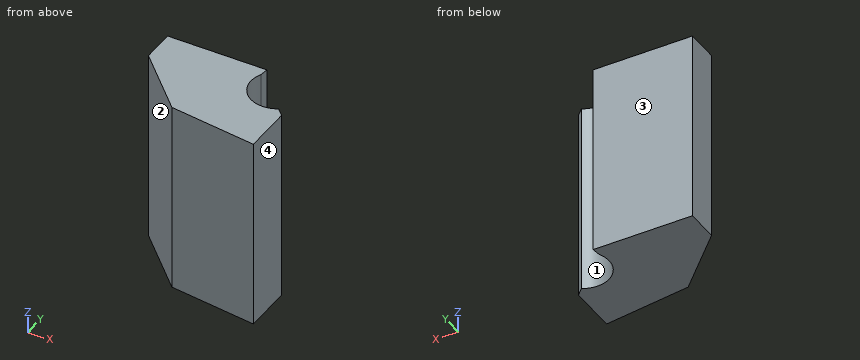
```python
from build123d import *

# Parameters (mm, degrees)
BOSS_EXTRU_1_DEPTH = 60
CHANFREIN1_START   = -1
CHANFREIN1_DEPTH   = 62
CHANFREIN2_SIZE    = 15
CHANFREIN2_SIZE2   = 17.409920551


with BuildPart() as part:
    # Esquisse1 → Boss.-Extru.1 (new body)
    with BuildSketch(Plane.XY):
        with BuildLine():
            Line((-1.739730228, 1.739730228), (-46.4022226, 7.592964471))
            Line((-46.4022226, 7.592964471), (-46.4022226, 32.915406071))
            Line((-46.4022226, 32.915406071), (-13.716955803, 32.915406071))
            ThreePointArc((-13.716955803, 32.915406071), (-14.250137868, 20.404998431), (-1.739730228, 20.938180496))
            Line((-1.739730228, 20.938180496), (-1.739730228, 1.739730228))
        make_face()
    extrude(amount=BOSS_EXTRU_1_DEPTH)

    # Chanfrein1: read off the stored shape, not the designer's step
    # Chanfrein1 outline → Chanfrein1 (cut)
    with BuildSketch(Plane.XY.offset(CHANFREIN1_START)):
        with BuildLine():
            ThreePointArc((-1.739730228, 20.938180496), (-2.7453552, 19.929895832), (-3.905196789, 19.103647058))
            Line((-3.905196789, 19.103647058), (-1.739730228, 16.938180496))
            Line((-1.739730228, 16.938180496), (-1.739730228, 20.938180496))
        make_face()
        with BuildLine():
            Line((-15.530475388, 32.915406071), (-15.835720777, 30.229973881))
            ThreePointArc((-15.835720777, 30.229973881), (-14.912820327, 31.680372218), (-13.716955803, 32.915406071))
            Line((-13.716955803, 32.915406071), (-15.530475388, 32.915406071))
        make_face()
    extrude(amount=CHANFREIN1_DEPTH, mode=Mode.SUBTRACT)

    # Chanfrein2
    chanfrein2_edges = [part.edges().sort_by_distance(p)[0] for p in [
        (-46.4022226, 7.592964471, 30),
    ]]
    chanfrein2_side = [part.faces().sort_by_distance(p)[0] for p in [
        (-46.4022226, 20.254185271, 30),
    ]]
    chamfer(chanfrein2_edges, length=CHANFREIN2_SIZE, length2=CHANFREIN2_SIZE2, reference=chanfrein2_side[0])


solid = part.part
```
The listing builds one solid part. Answer for the finished solid, in the listing's coordinates (mm). Face numbers are marked on the shaded views. Round coordinates to 2 decimals unless told otherwise and drop trailing zeros. Loops run counter-clockwise (first coordinate to the right, second up) from the corner with the lowest first, then second, coordinate; pieces in that order, holes last.
Q1. For a pull along Y with two mould halves and no side action, classify the marked faces 1, 2, 3 and 4 as released by +Y, released by -Y, zero draft, split by the parting line, or undercut.
Q2. Section A-A, the plane z = 49 is taken. Determine the outline of the cut face in (x, y), then the cut area to 3 significant figures.
Q3. Find the intervals of material crossed by line 1 (X direction, y = 7.5, z = 22.5); line 2 (Y direction, x = -45, z = 53.5); line 3 (Y direction, x = -37, z = 21), in increasing order.
Q4. Section B-B, the plane y = 27 is taken. Determine the outline of the cut face in (x, z).
Q5. Section C-C, the plane x = -22.5 is taken. Determine the outline of the cut face in (y, z).
Q6. Given pin 1 Ø8 at (y, z) = (23.5, 31.5) entering from +X; pin 2 Ø6 at (y, z) = (6.5, 13) entering from -X; pin 3 Ø3 at (x, z) = (-7, 15.5) entering from +Y, each flat-ended and moving along its own axis, determine where each tip first touches the part or whether it passes through.
Completed:
1. face 1: undercut
1. face 2: released by -Y
1. face 3: released by +Y
1. face 4: zero draft
2. outline: (-46.4, 22.59) - (-29.14, 5.33) - (-1.74, 1.74) - (-1.74, 16.94) - (-3.91, 19.1) arc R8.5 cw to (-15.84, 30.23) - (-15.53, 32.92) - (-46.4, 32.92) - close
2. area: 929 mm2
3. line 1: x = -31.31 to -1.74
3. line 2: y = 21.19 to 32.92
3. line 3: y = 13.19 to 32.92
4. outline: (-46.4, 0) - (-16.72, 0) - (-16.72, 60) - (-46.4, 60) - close
5. outline: (4.46, 0) - (32.92, 0) - (32.92, 60) - (4.46, 60) - close
6. pin 1: stops at x = -13.18
6. pin 2: stops at x = -33.31
6. pin 3: stops at y = 18.37
